The figure shows three views and two pictorial views of one solid part (mm, origin at its lowest corner). Answer the questions. A direction names the side the tool comes from. Coordinates: 2 decimals unless noted, no trailing zeros. Loops run counter-clockwise (first coordinate to the right, second up) from the corner with the lowest first, then second, coordinate; pieces in that order, holes last. Notation, with made-up numbers: (87.25, 23) - (104.25, 23) arc R14 cw to (104.25, 37) - close; hole circle Ø9 at (40.5, 49.25). An arc over 180 degrees is marked (long way). Write each question's results on one line, items separated by ' | '. Start each with the question number.
Item 1: Section A-A, the plane y = 13.5 is taken. Write down the section's boundary in (x, z), plus the area to 3 significant figures.
Item 2: Section B-B, the plane z = 16 is taken. Write down the section's boundary in (x, y).
Item 3: Section D-D, the plane z = 9 is taken. Write down the section's boundary in (x, y).
Item 4: Consider probe 1 along X at (y, z) = (0.95, 9); probe 2 along X at (y, z) = (5, 9); probe 3 along Z at (x, y) = (17, 10). Determine where each line is inside the solid, lowest interval first. Write a range as [from, to].
Item 5: A tool of negligible diameter and unlimited length cuts with its end or side. For the marked faces 4, 5, 6 and 7, from which of +Z, -Z, +X, -X, +Y, -Y can it reach the whole face along a straight path? Write none if from no direction.
Item 6: Section C-C, the plane x = 11 is taken. Write down the section's boundary in (y, z).
Item 7: For a pull along Y with two mould halves and no side action, classify the marked faces 1, 2 and 3 as +Y half, -Y half, draft (parallel to the pull), parting line (faces both ways), or undercut.
Item 8: Each of these flat-tipped pins is pushed along its axis until it touches: pin 1 Ø3 at (y, z) = (13, 11) entering from -X; pin 2 Ø1.5 at (x, z) = (10, 9.5) entering from +Y; pin 3 Ø2.5 at (x, z) = (11, 9) entering from +Y; pin 4 Ø5.5 at (x, y) = (3, 10) entering from +Z. Where does it stop, or does it pass through?
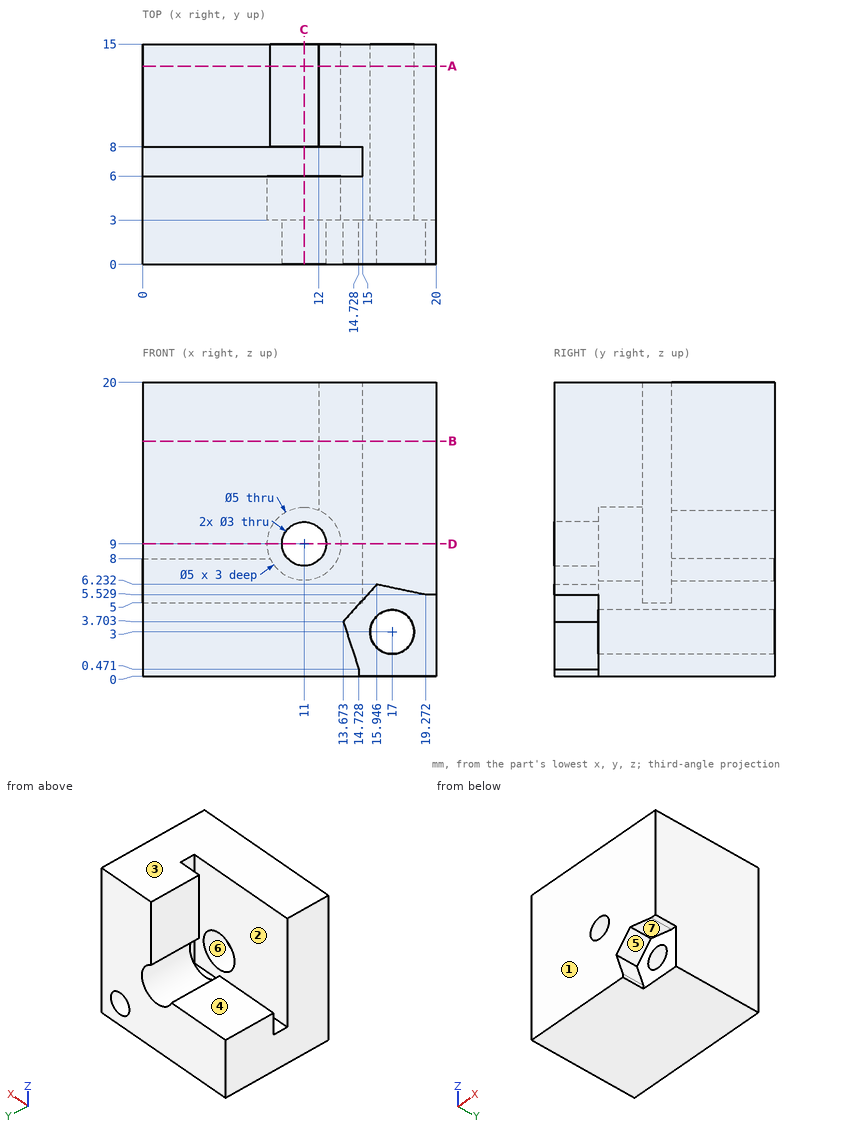
Answer key:
1) outline: (0, 0) - (20, 0) - (20, 20) - (12, 20) - (12, 11.29) arc R2.5 cw (long way) to (8.71, 8) - (0, 8) - close; hole circle Ø3 at (17, 3) | area: 240 mm^2
2) outline: (0, 0) - (20, 0) - (20, 15) - (12, 15) - (12, 8) - (15, 8) - (15, 6) - (0, 6) - close
3) outline: (0, 0) - (9.5, 0) - (9.5, 3) - (8.5, 3) - (8.5, 6) - (0, 6) - close; (12.5, 0) - (20, 0) - (20, 15) - (13.5, 15) - (13.5, 8) - (15, 8) - (15, 6) - (13.5, 6) - (13.5, 3) - (12.5, 3) - close
4) probe 1: x = [0, 9.5], [12.5, 20] | probe 2: x = [0, 8.5], [13.5, 20] | probe 3: z = [0, 1.5], [4.5, 20]
5) face 4: +Z, -X, +Y | face 5: -Y | face 6: +Y | face 7: -Z, -Y
6) outline: (0, 0) - (15, 0) - (15, 6.5) - (8, 6.5) - (8, 5) - (6, 5) - (6, 6.5) - (3, 6.5) - (3, 7.5) - (0, 7.5) - close; (0, 10.5) - (3, 10.5) - (3, 11.5) - (6, 11.5) - (6, 20) - (0, 20) - close
7) face 1: -Y half | face 2: undercut | face 3: draft
8) pin 1: stops at x = 12 | pin 2: stops at y = 3 | pin 3: passes through | pin 4: stops at z = 8
